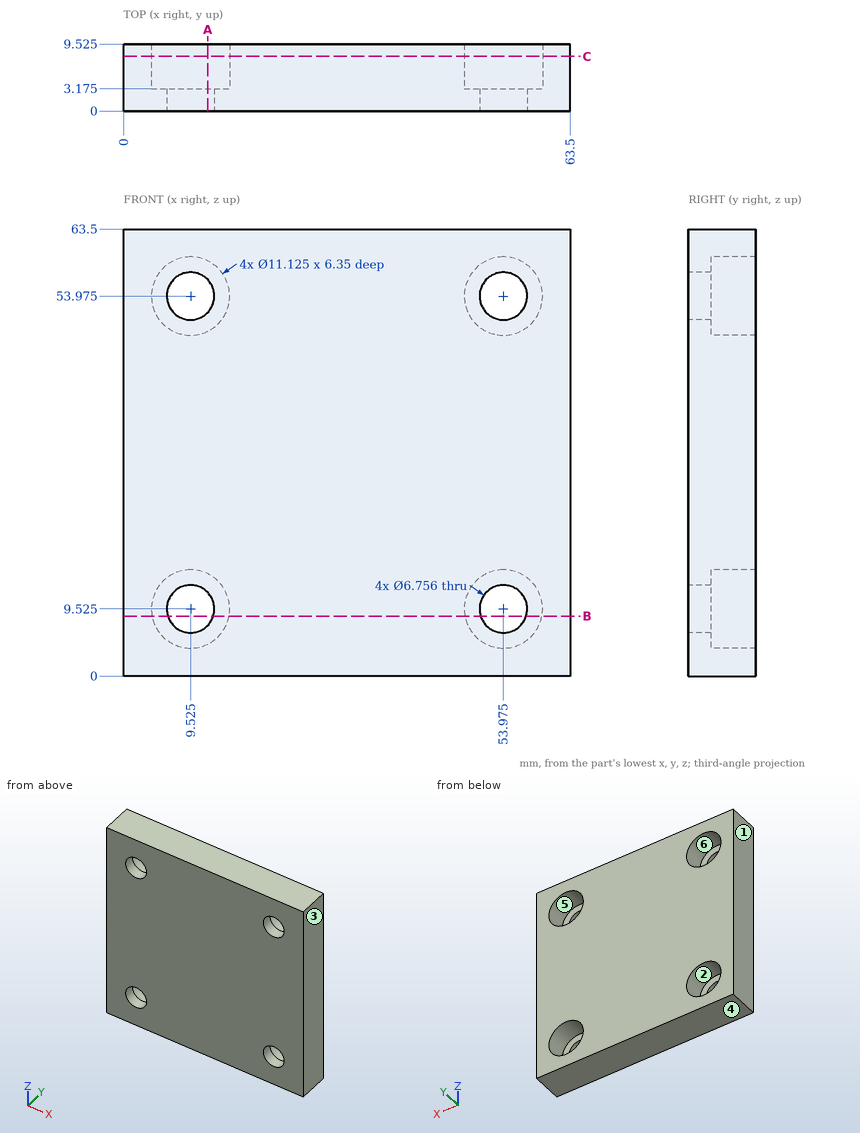
Job drawing, mm, ordinate dimensions from the low corner. One solid piece. A direction names the side the tool comes from. Round coordinates to 2 decimals unless told otherwise and drop trailing zeros. Write each loop counter-clockwise with the first axis right and the second up, starting at its lowest first coordinate (ties: lowest second). Pieces come first, ordered by that corner, then holes.
1) Band-saw the part on B-B, the plane z = 8.5. List the corners of the cut face in (x, y) (1 decimal), and give its area (3 significant figures).
2) Pin check, flat tips, straight feed: pin 1 (5.5 mm diameter, centred on x = 51.5, z = 53, fed in from +Y) (3 decimals); pin 2 (5.5 mm diameter, centred on x = 53.975, z = 9.525, fed in from +Y). Stop position of each tip, or through.
3) Drill centre lines: probe 1 along Z at (x, y) = (54, 6); probe 2 along X at (y, z) = (2, 55) (1 decimal); probe 3 along Z at (x, y) = (11.5, 2) (1 decimal). Where is each one in solid material? Low to high.
4) 3-axis set-ups, long thin cutter, end or side, ignore diameter. For the marked faces 1 and 2: which of +Z, -Z, +X, -X, +Y, -Y reach the whole face in a straight line?
5) Band-saw the part on C-C, the plane y = 7.75. List the corners of the cut face in (x, z) (1 decimal).
6) Band-saw the part on A-A, the plane x = 12. List the corners of the cut face in (y, z) (1 decimal), and give its area (3 significant figures).
7) Mould opens along X. For the marked faces 3, 4, 5 and 6 say: +X half, -X half, draft (parallel to the pull), parting line (faces both ways), or undercut.
Ans:
1. outline: (0, 0) - (6.3, 0) - (6.3, 3.2) - (4.1, 3.2) - (4.1, 9.5) - (0, 9.5) - close; (12.7, 0) - (50.8, 0) - (50.8, 3.2) - (48.5, 3.2) - (48.5, 9.5) - (15, 9.5) - (15, 3.2) - (12.7, 3.2) - close; (57.2, 0) - (63.5, 0) - (63.5, 9.5) - (59.4, 9.5) - (59.4, 3.2) - (57.2, 3.2) - close
1. area: 425 mm2
2. pin 1: stops at y = 3.175
2. pin 2: passes through
3. probe 1: z = 0 to 3.96, 15.09 to 48.41, 59.54 to 63.5
3. probe 2: x = 0 to 6.3, 12.7 to 50.8, 57.2 to 63.5
3. probe 3: z = 0 to 6.8, 12.3 to 51.2, 56.7 to 63.5
4. face 1: +Z, -Z, -X, +Y, -Y
4. face 2: +Y
5. outline: (0, 0) - (63.5, 0) - (63.5, 63.5) - (0, 63.5) - close; hole circle Ø11.1 at (9.5, 9.5); hole circle Ø11.1 at (9.5, 54); hole circle Ø11.1 at (54, 9.5); hole circle Ø11.1 at (54, 54)
6. outline: (0, 0) - (9.5, 0) - (9.5, 4.5) - (3.2, 4.5) - (3.2, 7.2) - (0, 7.2) - close; (0, 11.8) - (3.2, 11.8) - (3.2, 14.5) - (9.5, 14.5) - (9.5, 49) - (3.2, 49) - (3.2, 51.7) - (0, 51.7) - close; (0, 56.3) - (3.2, 56.3) - (3.2, 59) - (9.5, 59) - (9.5, 63.5) - (0, 63.5) - close
6. area: 449 mm2
7. face 3: +X half
7. face 4: draft
7. face 5: undercut
7. face 6: undercut
